Read the model definition and answer for the solid it produces. Units are mm, in the model's axes. Face numbers are marked on the shaded views. A direction names the side the tool comes from. Round coordinates to 2 decimals unless told otherwise and drop trailing zeros. Loops run counter-clockwise (first coordinate to the right, second up) from the corner with the lowest first, then second, coordinate; pieces in that order, holes last. Notation, with made-up numbers: (61, -15) - (85, -15) arc R31 ccw to (85, 21) - close; hole circle Ø8 at (34, 84). An arc over 180 degrees is marked (long way). Use one line per item in the form item = value. Start each with the question number.
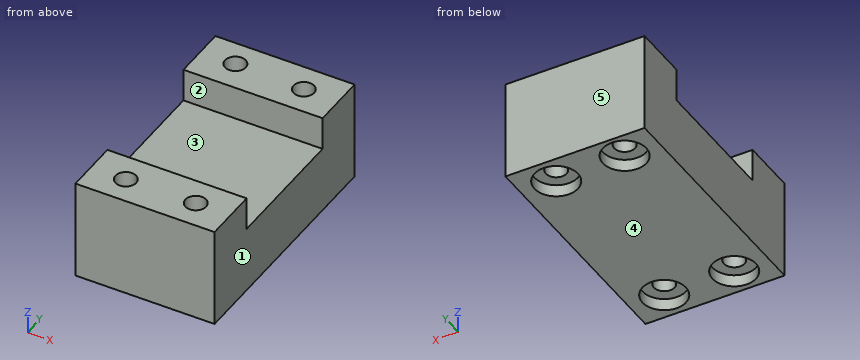
```python
from build123d import *

# Parameters (mm, degrees)
SKETCH1_W                                           = 25.4
SKETCH1_H                                           = 44.45
BOSS_EXTRUDE2_DEPTH                                 = 18.288
SKETCH3_W                                           = 25.4
SKETCH3_H                                           = 24.13
CUT_EXTRUDE1_DEPTH                                  = 6.096
CBORE_FOR_6_BINDING_HEAD_MACHINE_SCREW1_D           = 3.7973
CBORE_FOR_6_BINDING_HEAD_MACHINE_SCREW1_CBORE_D     = 7.9375
CBORE_FOR_6_BINDING_HEAD_MACHINE_SCREW1_CBORE_DEPTH = 2.2098


with BuildPart() as part:
    # Sketch1 → Boss-Extrude2 (new body)
    with BuildSketch(Plane.XY):
        with Locations((12.7, 22.225)):
            Rectangle(SKETCH1_W, SKETCH1_H)
    extrude(amount=BOSS_EXTRUDE2_DEPTH)

    # Sketch3 → Cut-Extrude1 (cut)
    with BuildSketch(Plane.XY.offset(18.288)):
        with Locations((12.7, 22.225)):
            Rectangle(SKETCH3_W, SKETCH3_H)
    extrude(amount=-CUT_EXTRUDE1_DEPTH, mode=Mode.SUBTRACT)

    # CBORE for #6 Binding Head Machine Screw1 (through all)
    with Locations(Plane(origin=(19.05, 5.08, 0), x_dir=(-1, 0, 0), z_dir=(0, 0, -1))):
        with Locations((0, 0), (12.699317265, -0.131685219), (0, 34.29), (12.694984111, 34.646901144)):
            CounterBoreHole(CBORE_FOR_6_BINDING_HEAD_MACHINE_SCREW1_D / 2, CBORE_FOR_6_BINDING_HEAD_MACHINE_SCREW1_CBORE_D / 2, CBORE_FOR_6_BINDING_HEAD_MACHINE_SCREW1_CBORE_DEPTH)


solid = part.part
```
1) Flat-ended cylindrical pins translate along their axes: pin 1 (2.5 mm diameter, centred on x = 5.5, y = 5.5, fed in from -Z); pin 2 (2.5 mm diameter, centred on x = 18.5, y = 5, fed in from -Z). Find the tip coordinate at first contact, or state that the pin passes through.
2) A cutting plane is placed at B-B on x = 19.05. Write down the section's boundary in (y, z).
3) Straight lines are drawn through the part: line 1 (Y direction, x = 19.05, z = 0.7); line 2 (Y direction, x = 11.75, z = 16.5); line 3 (Y direction, x = 19.05, z = 12.5). For each, find the intervals that lie inside material, in ascending order. Write a range as from..to.
4) A cutting plane is placed at D-D on z = 8.75. Write down the section's boundary in (x, y), plus the area to 3 significant figures.
5) Determine the mould class of the marked faces 3, 4 and 5 for opening direction Y: +Y half, -Y half, draft (parallel to the pull), parting line (faces both ways), or undercut.
6) For the marked faces 1 and 2, determine the directions among +Z, -Z, +X, -X, +Y, -Y from which every point of the face is accessible in a straight line to the end or side of a thin tool.
7) A cutting plane is placed at C-C on y = 4.5. Write down the section's boundary in (x, z).
8) A cutting plane is placed at A-A on z = 16.5. Write down the section's boundary in (x, y).
Checks:
q1.pin_1 = 2.21
q1.pin_2 = through
q2.outline = (0, 0) - (1.11, 0) - (1.11, 2.21) - (3.18, 2.21) - (3.18, 18.29) - (0, 18.29) - close; (6.98, 2.21) - (9.05, 2.21) - (9.05, 0) - (35.4, 0) - (35.4, 2.21) - (37.47, 2.21) - (37.47, 18.29) - (34.29, 18.29) - (34.29, 12.19) - (10.16, 12.19) - (10.16, 18.29) - (6.98, 18.29) - close; (41.27, 2.21) - (43.34, 2.21) - (43.34, 0) - (44.45, 0) - (44.45, 18.29) - (41.27, 18.29) - close
q3.line_1 = 0..1.11, 9.05..35.4, 43.34..44.45
q3.line_2 = 0..10.16, 34.29..44.45
q3.line_3 = 0..3.18, 6.98..10.16, 34.29..37.47, 41.27..44.45
q4.outline = (0, 0) - (25.4, 0) - (25.4, 44.45) - (0, 44.45) - close; hole circle Ø3.8 at (6.35, 4.95); hole circle Ø3.8 at (6.36, 39.73); hole circle Ø3.8 at (19.05, 5.08); hole circle Ø3.8 at (19.05, 39.37)
q4.area = 1,080 mm²
q5.face_3 = undercut
q5.face_4 = draft
q5.face_5 = +Y half
q6.face_1 = +Z, -Z, +X, +Y, -Y
q6.face_2 = +Z, +X, -X
q7.outline = (0, 0) - (2.41, 0) - (2.41, 2.21) - (4.51, 2.21) - (4.51, 18.29) - (0, 18.29) - close; (8.2, 2.21) - (10.29, 2.21) - (10.29, 0) - (15.12, 0) - (15.12, 2.21) - (17.24, 2.21) - (17.24, 18.29) - (8.2, 18.29) - close; (20.86, 2.21) - (22.98, 2.21) - (22.98, 0) - (25.4, 0) - (25.4, 18.29) - (20.86, 18.29) - close
q8.outline = (0, 0) - (25.4, 0) - (25.4, 10.16) - (0, 10.16) - close; (0, 34.29) - (25.4, 34.29) - (25.4, 44.45) - (0, 44.45) - close; hole circle Ø3.8 at (6.35, 4.95); hole circle Ø3.8 at (6.36, 39.73); hole circle Ø3.8 at (19.05, 5.08); hole circle Ø3.8 at (19.05, 39.37)
